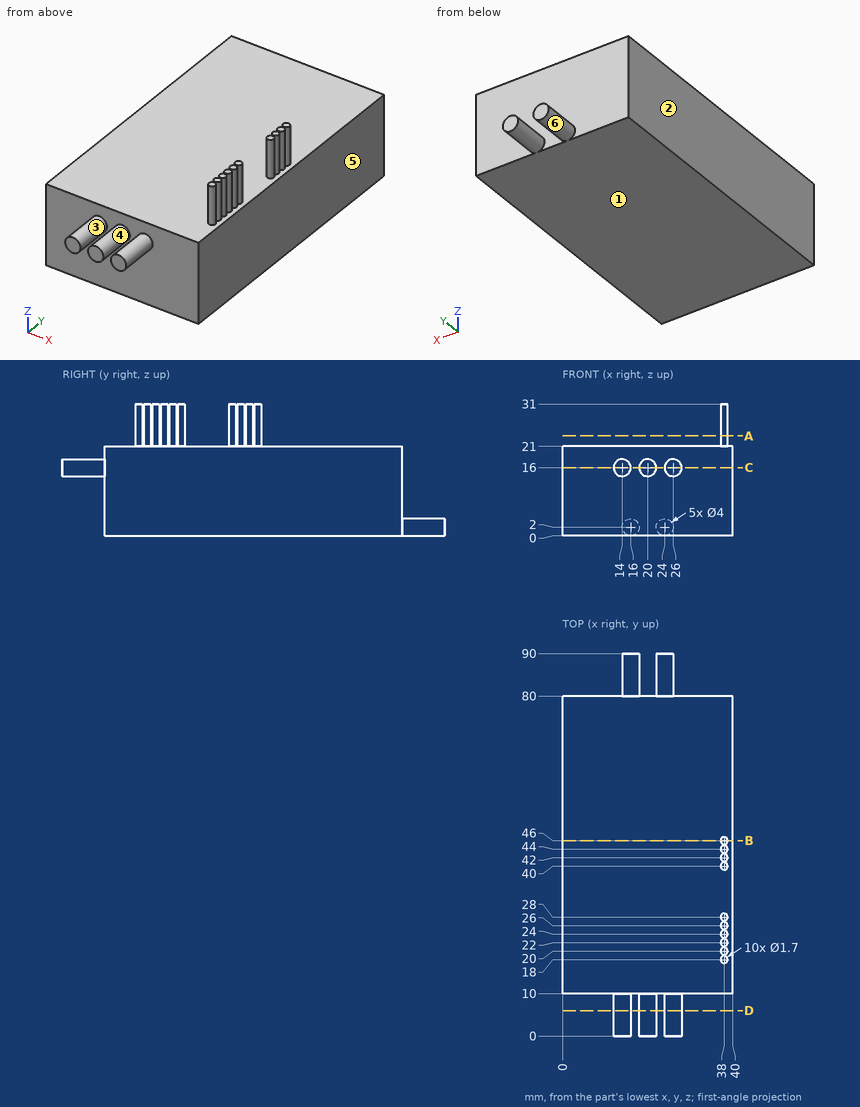
Geometry: see drawing. Coordinates: mm, zero at the bounding-box minimum. A direction names the side the tool comes from. Coordinates: 2 decimals unless noted, no trailing zeros. Loops run counter-clockwise (first coordinate to the right, second up) from the corner with the lowest first, then second, coordinate; pieces in that order, holes last. Notation, with made-up numbers: M -14,-33 L 25,-33 A9 ccw 25,-21 Z; hole C 28,-26.5 d10. An arc over 180 degrees is marked long. Put each result on its own line as item: value. Start each with the question number.
1) Reachability of the marked faces 4, 5 and 6 from +Z, -Z, +X, -X, +Y, -Y: full face, straight path, thin tool, end or side. Return the list, or none.
2) Cut plane C-C on z = 16. Return the cut outline in (x, y).
3) Contact query for flat-ended pins moving along their axis: pin 1 Ø12 at (x, y) = (23, 73.5) entering from +Z; pin 2 Ø8 at (x, z) = (8.5, 17.5) entering from +Y; pin 3 Ø5 at (x, z) = (14.5, 24) entering from +Y. Output: stop coordinate, or through.
4) Cut plane B-B on y = 46. Return the cut outline in (x, z).
5) Ray query, L1, parallel to Y at x = 8.5, z = 19.5; L2, parallel to Z at x = 15, y = 22.5; L3, parallel to X at y = 27.5, z = 28. Return the intervals inside material, ascending. Write a range as from..to.
6) Pull-direction query (X, two-part tool) for the marked faces 1, 2 and 3; classes: pulls with the +X half, pulls with the -X half, needs draft (parallel to the pull), parting line crosses it, or undercut.
7) Cut plane A-A on z = 23.5. Give the number of separate pieces and of enclosed holes in the cut face, then the cut area to 3 significant figures.
8) Cut plane D-D on y = 6. Return the cut outline in (x, z), then the cut area to 3 significant figures.
The answers:
1. face 4: -Y
1. face 5: +Z, -Z, +X, +Y, -Y
1. face 6: +Y
2. outline: M 0,10 L 12,10 L 12,0 L 16,0 L 16,10 L 18,10 L 18,0 L 22,0 L 22,10 L 24,10 L 24,0 L 28,0 L 28,10 L 40,10 L 40,80 L 0,80 Z
3. pin 1: stops at z = 21
3. pin 2: stops at y = 80
3. pin 3: passes through
4. outline: M 0,0 L 40,0 L 40,21 L 38.85,21 L 38.85,31 L 37.15,31 L 37.15,21 L 0,21 Z
5. L1: y = 10..80
5. L2: z = 0..21
5. L3: x = 37.31..38.69
6. face 1: needs draft
6. face 2: pulls with the -X half
6. face 3: undercut
7. separate pieces: 10
7. enclosed holes: 0
7. area: 22.7 mm²
8. outline: C 14,16 d4; C 20,16 d4; C 26,16 d4
8. area: 37.7 mm²
